For this review, take the finished solid that the model builds, in its own axes (mm). A direction names the side the tool comes from. Round coordinates to 2 decimals unless told otherwise and drop trailing zeros. Order: outer loops, then holes, each group sorted by start corner. A loop starts at its lowest first (then second) coordinate and runs counter-clockwise, first axis right, second up. Notation, with made-up numbers: M -38,29.5 L -30,29.5 A19 ccw -30,65.5 Z; hole C -15.75,24.25 d1. An arc over 180 degrees is marked long. Put each result on its own line as item: value.
from build123d import *

# Parameters (mm, degrees)
SKETCH4_W                = 85.972725278
SKETCH4_H                = 1
EXTRUDE_THIN1_DEPTH      = 0.5
SKETCH6_R                = 5
CUT_EXTRUDE1_DEPTH       = 10
BOSS_EXTRUDE2_DEPTH      = 0.5
BOSS_EXTRUDE2_DEPTH_BACK = 5
SKETCH7_R                = 3.739985504
BOSS_EXTRUDE3_START      = -0.5
SKETCH8_R                = 5
SKETCH8_R_2              = 3
BOSS_EXTRUDE3_DEPTH      = 1
MOVE_FACE1_BY            = 2
SKETCH10_R               = 3.589046815
CUT_EXTRUDE4_DEPTH       = 1
MOVE_FACE2_BY            = 5
SKETCH11_R               = 5
SKETCH11_R_2             = 3.589046815
BOSS_EXTRUDE4_DEPTH      = 2.93


with BuildPart() as part:
    # Sketch4 → Extrude-Thin1 (new, symmetric)
    with BuildSketch(Plane.XY):
        with Locations((71.721545049, 0)):
            Rectangle(SKETCH4_W, SKETCH4_H)
    extrude(amount=EXTRUDE_THIN1_DEPTH, both=True)

    # Sketch6 → Cut-Extrude1 (cut)
    with BuildSketch(Plane.XY.offset(0.5)):
        with Locations((28.73518241, 0)):
            Circle(SKETCH6_R)
    extrude(amount=-CUT_EXTRUDE1_DEPTH, mode=Mode.SUBTRACT)

    # Sketch7 → Boss-Extrude2 (add, two sides: drawn at the far end of the back side and taken through both)
    with BuildSketch(Plane.XY.offset(-BOSS_EXTRUDE2_DEPTH_BACK)):
        with Locations(Location((114.707907688, 0, 0), (0, 0, 187.682896446))):
            Circle(SKETCH7_R)
    extrude(amount=BOSS_EXTRUDE2_DEPTH + BOSS_EXTRUDE2_DEPTH_BACK)

    # Sketch8 → Boss-Extrude3 (add)
    with BuildSketch(Plane.XY.offset(BOSS_EXTRUDE3_START)):
        with Locations((28.73518241, 0)):
            Circle(SKETCH8_R)
        with Locations((28.73518241, 0)):
            Circle(SKETCH8_R_2, mode=Mode.SUBTRACT)
    extrude(amount=BOSS_EXTRUDE3_DEPTH)

    # Move Face1: a face moved outward by 2.0
    extrude(part.faces().sort_by_distance((114.707907688, 0, -5))[0], amount=MOVE_FACE1_BY, dir=(0, 0, -1))

    # Sketch10 → Cut-Extrude4 (cut)
    with BuildSketch(Plane.XY.offset(0.5)):
        with Locations((28.73518241, 0)):
            Circle(SKETCH10_R)
    extrude(amount=-CUT_EXTRUDE4_DEPTH, mode=Mode.SUBTRACT)

    # Move Face2: a face moved inward by 5.0
    extrude(part.faces().sort_by_distance((114.707907688, 0, -7))[0], amount=MOVE_FACE2_BY, dir=(0, 0, 1), mode=Mode.SUBTRACT)

    # Sketch11 → Boss-Extrude4 (add)
    with BuildSketch(Plane(origin=(0, 0, -0.5), x_dir=(-1, 0, 0), z_dir=(0, 0, -1))):
        with Locations((-28.73518241, 0)):
            Circle(SKETCH11_R)
        with Locations(Location((-28.73518241, 0, 0), (0, 0, 180))):
            Circle(SKETCH11_R_2, mode=Mode.SUBTRACT)
    extrude(amount=BOSS_EXTRUDE4_DEPTH)


solid = part.part
(1) To check wall thickness, follow L1, parallel to X at y = -3, z = -0.2; L2, parallel to X at y = 2, z = 0.3; L3, parallel to X at y = 0.25, z = -3. State the ranges of each line that lie inside material, in increasing order.
A:
L1: x = 24.74 to 26.77, 30.71 to 32.74, 112.47 to 116.94
L2: x = 24.15 to 25.76, 31.72 to 33.32, 111.55 to 117.87
L3: x = 23.74 to 25.15, 32.32 to 33.73
(2) Add section A-A on z = -1.15. Give the boundary of the cut face in (x, y), then the cut area to 3 significant figures.
A:
outline: C 28.74,0 d10; C 114.71,0 d7.48; hole C 28.74,0 d7.18
area: 82.0 mm2
(3) For faces 1 (the face through (115, 0, -2)), 2 (the face through (71, 0, 0.5)), list the 3-axis set-ups (+Z, -Z, +X, -X, +Y, -Y) from which the entire face can be reached by the end or side of a thin tool; tool diameter is ignored.
A:
face 1: -Z, +X, +Y, -Y
face 2: +Z, +X, -X, +Y, -Y
(4) Draft analysis for pull direction X (two halves, no side actions). For faces 3 (the face through (118.433, 0.337, -0.768)), 4 (the face through (25, -2, -3.43)), state which applies: released by +X, released by -X, zero draft, split by the parting line, or undercut.
A:
face 3: undercut
face 4: zero draft
(5) Insertion check: pin 1 Ø1.5 at (x, z) = (82.5, 0) entering from -Y; pin 2 Ø4.5 at (x, y) = (28.74, 0) entering from +Z; pin 3 Ø1.1 at (x, z) = (77, 0) entering from +Y; pin 4 Ø6 at (x, y) = (115, 0.5) entering from -Z. Each pin has a flat end and moves straight along its axis. Give the tip position at first contact, or say it passes through.
A:
pin 1: stops at y = -0.5
pin 2: passes through
pin 3: stops at y = 0.5
pin 4: stops at z = -2
(6) Add section B-B on y = 1.5. Give the boundary of the cut face in (x, z), then the cut area to 3 significant figures.
A:
outline: M 23.97,-3.43 L 25.47,-3.43 L 25.47,0.5 L 23.97,0.5 Z; M 32,-3.43 L 33.5,-3.43 L 33.5,0.5 L 32,0.5 Z; M 111.28,-2 L 118.13,-2 L 118.13,0.5 L 111.28,0.5 Z
area: 29.0 mm2
(7) Add section C-C on x = 77. Give the boundary of the cut face in (y, z).
A:
outline: M -0.5,-0.5 L 0.5,-0.5 L 0.5,0.5 L -0.5,0.5 Z
